Design review of the part shown in the three views and the two pictorial views. Dimensions are in mm from the part's minimum x, y and z. Round coordinates to 2 decimals unless told otherwise and drop trailing zeros. Loops run counter-clockwise (first coordinate to the right, second up) from the corner with the lowest first, then second, coordinate; pieces in that order, holes last.
1) Take a section at C-C (y = 0.95). Give the number of separate pieces and of enclosed holes in the cut face, then the cut area to 3 significant figures.
2) Wall thickness on L1, parallel to X at y = 0.75, z = 4; L2, parallel to Z at x = 19, y = 1.75; L3, parallel to Z at x = 18, y = 0.9: over which ranges is each line inside the solid? List them lowest first.
3) Take a section at A-A (z = 21.5). State the section outline as (x, y) points.
4) Insertion check: pin 1 (2.5 mm diameter, centred on x = 18, z = 4, fed in from -Y). The pin has a flat end and moves straight along its axis. Give the tip position at first contact, or say it passes through.
5) Take a section at D-D (z = 15). State the section outline as (x, y) points, then the cut area to 3 significant figures.
6) Take a section at B-B (x = 9.25). State the section outline as (y, z) points.
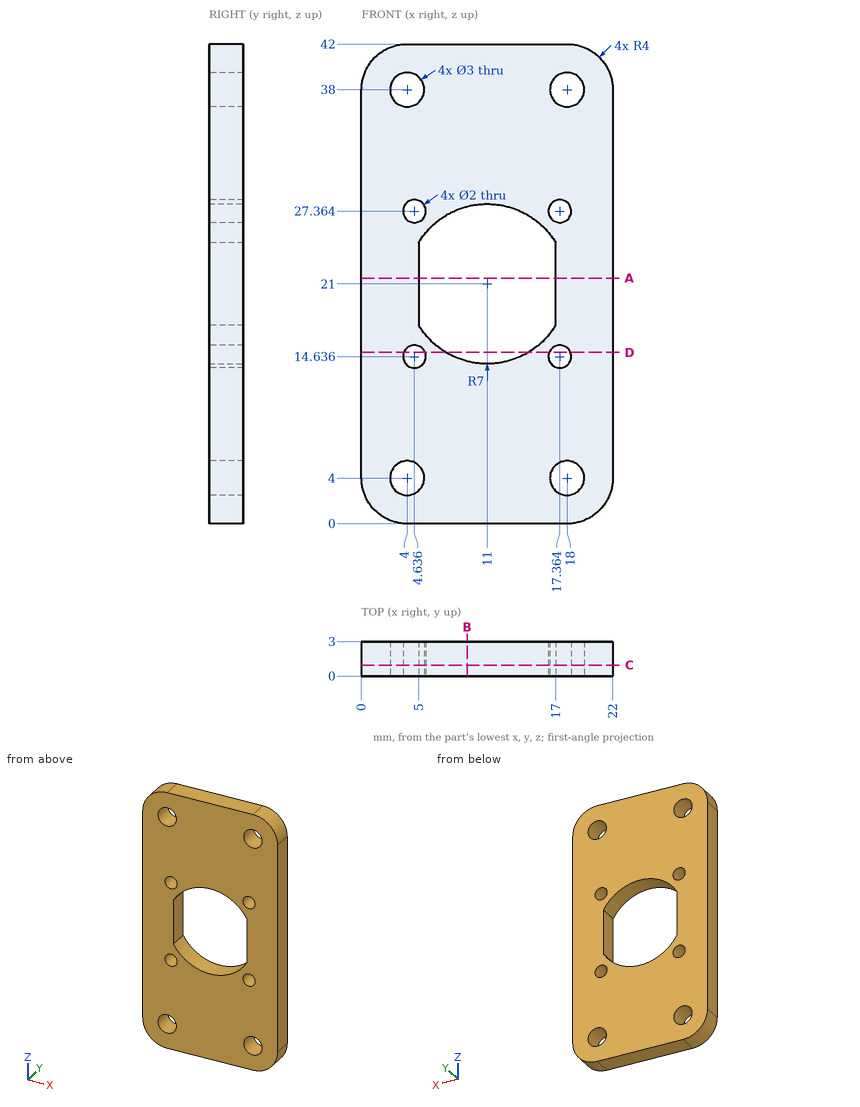
Response:
1. separate pieces: 1
1. enclosed holes: 9
1. area: 725 mm2
2. L1: x = 0 to 2.5, 5.5 to 16.5, 19.5 to 22
2. L2: z = 0.13 to 2.88, 5.12 to 36.88, 39.12 to 41.87
2. L3: z = 0 to 2.5, 5.5 to 13.86, 15.41 to 26.59, 28.14 to 36.5, 39.5 to 42
3. outline: (0, 0) - (5, 0) - (5, 3) - (0, 3) - close; (17, 0) - (22, 0) - (22, 3) - (17, 3) - close
4. pin 1: passes through
5. outline: (0, 0) - (3.7, 0) - (3.7, 3) - (0, 3) - close; (5.57, 0) - (7.39, 0) - (7.39, 3) - (5.57, 3) - close; (14.61, 0) - (16.43, 0) - (16.43, 3) - (14.61, 3) - close; (18.3, 0) - (22, 0) - (22, 3) - (18.3, 3) - close
5. area: 33.2 mm2
6. outline: (0, 0) - (3, 0) - (3, 14.22) - (0, 14.22) - close; (0, 27.78) - (3, 27.78) - (3, 42) - (0, 42) - close
